Work out the finished part from the listing and answer in its coordinate system (mm). Round coordinates to 2 decimals unless told otherwise and drop trailing zeros. Write each loop counter-clockwise with the first axis right and the second up, starting at its lowest first coordinate (ties: lowest second). Pieces come first, ordered by that corner, then holes. Notation, with made-up numbers: M -37.75,65.25 L 1.25,65.25 A11 cw 1.25,79.25 Z; hole C 36,38.25 d6. An arc over 180 degrees is marked long. One line per item, written item: value. Start each with the question number.
Q1. The mould has two halves that part along Z. Classify faces 1 (the cylindrical face through (4.48, 0.72, 13.02)), 2 (the flat face through (5.69, 8.1, -1)), 3 (the cylindrical face through (4.483, 5.891, -11.634)), 4 (the cylindrical face through (4.488, 12.932, 5.362)): released by +Z, released by -Z, zero draft, split by the parting line, or undercut.
Q2. Consider probe 1 along Z at (x, y) = (5.1, 6.5); probe 2 along Y at (x, z) = (4.6, 6); probe 3 along Y at (x, z) = (5.25, 5) (3 decimals). Determine where each line is inside the solid, lowest interval first.
Q3. Find section A-A (z = 0). Write down the section's boundary in (x, y).
Q4. Given pin 1 Ø1 at (x, y) = (3.5, 2.5) entering from -Z; pin 2 Ø1 at (x, y) = (4, -1.5) entering from -Z; pin 3 Ø1 at (x, z) = (4, 7.5) entering from +Y, each flat-ended and moving along its own axis, determine where each tip first touches the part or whether it passes through.
Q5. Find section B-B (x = 4.9). Count the separate pieces of the cut face and the enclosed holes in it, and give its area (3 significant figures).
Autodesk Inventor part; units mm, degrees
ref_plane "YZ Plane" through (0, 0, 0) normal (1, 0, 0) x (0, 1, 0)
ref_plane "XZ Plane" through (0, 0, 0) normal (0, 1, 0) x (-1, 0, 0)
ref_plane "XY Plane" through (0, 0, 0) normal (0, 0, 1) x (1, 0, 0)
sketch "Sketch_1" plane through (0, 0, 0) normal (0, 0, 1) x (1, 0, 0)
  line L0 (5.6905, 0) -> (3.3095, 0)
  line L1 (3.3095, 13.7) -> (3.3095, 8)
  line L2 (3.3095, 8) -> (5.6905, 8)
  line L3 (5.6905, 8) -> (5.6905, 13.7)
  arc A0 (5.6905, 13.7) -> (5.3905, 14) centre (5.3905, 13.7) ccw
  line L4 (5.3905, 14) -> (3.6095, 14)
  arc A1 (3.6095, 14) -> (3.3095, 13.7) centre (3.6095, 13.7) ccw
revolve "Revolution1" add sketch "Sketch_1" angle 360 about axis through (5.6905, 0, 0) along (1, 0, 0)
sketch "Sketch_2" plane through (0, 0, 0) normal (1, 0, 0) x (0, 1, 0)
  circle A0 centre (10.75, 0) radius 2.381
extrude "Extrusion1" cut sketch "Sketch_2" along normal blind 9
pattern_circular "Circular Pattern1" count 12 over 360 about axis through (0, 0, 0) along (1, 0, 0) of "Extrusion1"
properties part number "SKF_51102_PART1"
The answers:
1. face 1: undercut
1. face 2: zero draft
1. face 3: undercut
1. face 4: split by the parting line
2. probe 1: -12.4 to -11.41, -7.21 to -4.66, 4.66 to 7.21, 11.41 to 12.4
2. probe 2: -12.65 to -11.61, -7.01 to -5.29, 5.29 to 7.01, 11.61 to 12.65
2. probe 3: -13.077 to -11.661, -6.958 to -6.245, 6.245 to 6.958, 11.661 to 13.077
3. outline: M 3.31,-13.7 A0.3 ccw 3.61,-14 L 5.39,-14 A0.3 ccw 5.69,-13.7 L 5.69,-13.13 L 3.31,-13.13 Z; M 3.31,-8.37 L 5.69,-8.37 L 5.69,-8 L 3.31,-8 Z; M 3.31,8 L 5.69,8 L 5.69,8.37 L 3.31,8.37 Z; M 3.31,13.13 L 5.69,13.13 L 5.69,13.7 A0.3 ccw 5.39,14 L 3.61,14 A0.3 ccw 3.31,13.7 Z
4. pin 1: z = -13.85
4. pin 2: z = -13.96
4. pin 3: y = 12.12
5. separate pieces: 1
5. enclosed holes: 13
5. area: 201 mm2
